Geometry: final body of the model. Coordinates: model frame, mm. Round coordinates to 2 decimals unless told otherwise and drop trailing zeros. Loops run counter-clockwise (first coordinate to the right, second up) from the corner with the lowest first, then second, coordinate; pieces in that order, holes last. Notation, with made-up numbers: (3, 10.25) - (24, 10.25) arc R8 ccw to (24, 19.25) - close; hole circle Ø5 at (81, -4). An arc over 180 degrees is marked (long way). Return JSON: item names as keys, results as strings. Group by question number.
1. Section D-D on y = -2.5. Return loops of the section in (x, z), and give its area (3 significant figures).
2. Section B-B on y = 2.25. Return loops of the section in (x, z), and give its area (3 significant figures).
3. First-contact query: pin 1 Ø3 at (x, y) = (0, 0) entering from -Z; pin 2 Ø2 at (y, z) = (2.5, 12.5) entering from +X. Flat tips, straight axial feed; report the tip coordinate or a pass-through.
4. Material intervals for probe 1 along Y at (x, z) = (0, -17.25) (3 decimals); probe 2 along Y at (x, z) = (-1, 26); probe 3 along X at (y, z) = (-0.75, 9), sorted ascending.
5. Section C-C on z = 6.5. Return loops of the section in (x, y) (3 decimals), and give its area (3 significant figures).
6. Section A-A on z = 15. Return loops of the section in (x, y) (3 decimals).
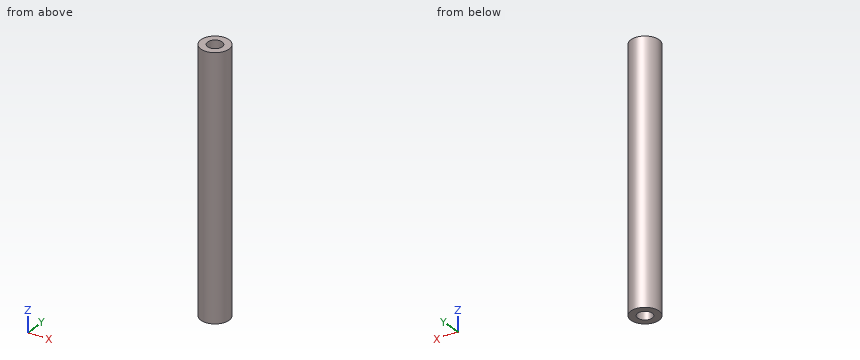
from build123d import *

# Parameters (mm, degrees)
SKETCH1_R           = 3.175
BOSS_EXTRUDE1_DEPTH = 29


with BuildPart() as part:
    # Sketch1 → Boss-Extrude1 (new, symmetric)
    with BuildSketch(Plane.XY):
        with Locations(Location((0, 0, 0), (0, 0, 180))):
            Circle(SKETCH1_R)
    extrude(amount=BOSS_EXTRUDE1_DEPTH, both=True)

    # Sketch3 → M4x0.7 Tapped Hole1 (revolve, cut)
    with BuildSketch(Plane(origin=(0, 0, 29), x_dir=(0, -1, 0), z_dir=(1, 0, 0))):
        Polygon((0, 0), (0, 18.009420021), (1.65, 17.018), (1.65, 0), align=None)
    m4x0_7_tapped_hole1 = revolve(axis=Axis((0, 0, 35.35), (0, 0, -1)), mode=Mode.SUBTRACT)

    # Mirror1: M4x0.7 Tapped Hole1 across plane
    add(m4x0_7_tapped_hole1.mirror(Plane.XY), mode=Mode.SUBTRACT)


solid = part.part
Taken from the geometry:
{
 "1": {"outline": "(-1.96, -29) - (1.96, -29) - (1.96, 29) - (-1.96, 29) - close", "area": "227 mm2"},
 "2": {"outline": "(-2.24, -29) - (2.24, -29) - (2.24, 29) - (-2.24, 29) - close", "area": "260 mm2"},
 "3": {"pin 1": "z = -11.89", "pin 2": "x = 2.8"},
 "4": {"probe 1": "-3.175 to -1.65, 1.65 to 3.175", "probe 2": "-3.01 to -1.31, 1.31 to 3.01", "probe 3": "-3.09 to 3.09"},
 "5": {"outline": "circle Ø6.35 at (0, 0)", "area": "31.7 mm2"},
 "6": {"outline": "circle Ø6.35 at (0, 0); hole circle Ø3.3 at (0, 0)"}
}
